Design review of the part built by this model. Coordinates are the model's own, in mm. A direction names the side the tool comes from. Coordinates: 2 decimals unless noted, no trailing zeros. Order: outer loops, then holes, each group sorted by start corner. A loop starts at its lowest first (then second) coordinate and runs counter-clockwise, first axis right, second up.
from build123d import *

# Parameters (mm, degrees)
SKETCH_1_R          = 1.6
EXTRUDE_1_DEPTH     = 3
SKETCH_2_R          = 1.6
CUT_EXTRUDE_1_DEPTH = 4
FILLET_1_R          = 3
SKETCH_4_R          = 1.6
CUT_EXTRUDE_2_DEPTH = 4
SKETCH_5_W          = 38
SKETCH_5_H          = 16
CUT_EXTRUDE_3_DEPTH = 4
FILLET_2_R          = 3


with BuildPart() as part:
    # 草图1 → 凸台-拉伸1 (new body)
    with BuildSketch(Plane.XY):
        Polygon((-40, 0), (-48, 25.544444444), (-48, 53.5), (5, 53.5), (5, 25.544444444), (0, 0), align=None)
        with Locations((-44, 49.5)):
            Circle(SKETCH_1_R, mode=Mode.SUBTRACT)
        with Locations((1, 49.5)):
            Circle(SKETCH_1_R, mode=Mode.SUBTRACT)
        with Locations((1, 27.5)):
            Circle(SKETCH_1_R, mode=Mode.SUBTRACT)
        with Locations((-44, 27.5)):
            Circle(SKETCH_1_R, mode=Mode.SUBTRACT)
    extrude(amount=EXTRUDE_1_DEPTH)

    # 草图2 → 切除-拉伸1 (cut, through all)
    with BuildSketch(Plane.XY.offset(3)):
        with Locations((-5, 3)):
            Circle(SKETCH_2_R)
        with Locations((-15, 3)):
            Circle(SKETCH_2_R)
        with Locations((-25, 3)):
            Circle(SKETCH_2_R)
        with Locations((-35, 3)):
            Circle(SKETCH_2_R)
    extrude(amount=-CUT_EXTRUDE_1_DEPTH, mode=Mode.SUBTRACT)

    # 圆角1
    fillet_1_edges = [part.edges().sort_by_distance(p)[0] for p in [
        (0, 0, 1.5),
        (-40, 0, 1.5),
        (-48, 25.544444444, 1.5),
        (-48, 53.5, 1.5),
        (5, 53.5, 1.5),
        (5, 25.544444444, 1.5),
    ]]
    fillet(fillet_1_edges, radius=FILLET_1_R)

    # 草图4 → 切除-拉伸2 (cut, through all)
    with BuildSketch(Plane.XY.offset(3)):
        with Locations((-21.5, 36.5)):
            Circle(SKETCH_4_R)
        with Locations((-33.5, 12.5)):
            Circle(SKETCH_4_R)
        with Locations((-21.5, 12.5)):
            Circle(SKETCH_4_R)
    extrude(amount=-CUT_EXTRUDE_2_DEPTH, mode=Mode.SUBTRACT)

    # 草图5 → 切除-拉伸3 (cut, through all)
    with BuildSketch(Plane(origin=(0, 0, 0), x_dir=(-1, 0, 0), z_dir=(0, 0, -1))):
        with Locations((21.5, 38.5)):
            Rectangle(SKETCH_5_W, SKETCH_5_H)
    extrude(amount=-CUT_EXTRUDE_3_DEPTH, mode=Mode.SUBTRACT)

    # 圆角2
    fillet_2_edges = [part.edges().sort_by_distance(p)[0] for p in [
        (-40.5, 46.5, 1.5),
        (-40.5, 30.5, 1.5),
        (-2.5, 30.5, 1.5),
        (-2.5, 46.5, 1.5),
    ]]
    fillet(fillet_2_edges, radius=FILLET_2_R)


solid = part.part
1. For faces 4 (the flat face through (-21, 27, 0)), 5 (the cylindrical face through (-39.64, 45.6, 1.52)), list the 3-axis set-ups (+Z, -Z, +X, -X, +Y, -Y) from which the entire face can be reached by the end or side of a thin tool; tool diameter is ignored.
2. Insertion check: pin 1 (3 mm diameter, centred on x = -25, y = 3, fed in from -Z). The pin has a flat end and moves straight along its axis. Give the tip position at first contact, or say it passes through.
3. To check wall thickness, follow line 1 (Y direction, x = -21.5, z = 1.2); line 2 (Y direction, x = -36, z = 2.3); line 3 (X direction, y = 36, z = 0.7). State the ranges of each line that lie inside material, in increasing order.
4. Add section B-B (x = -25). Give the boundary of the cut face in (y, z), and give its area (3 significant figures).
5. Mouldability with a two-part tool opening along Y and no side actions: class faces 1 (the cylindrical face through (-0.585, 0.666, 1.521)), 2 (the cylindrical face through (-3.4, 31.36, 1.52)), 3 (the flat face through (5, 38, 1)) as pulls with the +Y half, pulls with the -Y half, needs draft (parallel to the pull), parting line crosses it, or undercut.
6. Add section A-A (z = 1). State how many separate pieces and enclosed holes the cut face has, and give its area (3 significant figures).
Solution:
1. face 4: -Z, +X, -X, +Y, -Y
1. face 5: +Z, -Z
2. pin 1: passes through
3. line 1: y = 0 to 10.9, 14.1 to 30.5, 46.5 to 53.5
3. line 2: y = 0 to 1.75, 4.25 to 30.5, 46.5 to 53.5
3. line 3: x = -48 to -40.5, -2.5 to 5
4. outline: (0, 0) - (1.4, 0) - (1.4, 3) - (0, 3) - close; (4.6, 0) - (30.5, 0) - (30.5, 3) - (4.6, 3) - close; (46.5, 0) - (53.5, 0) - (53.5, 3) - (46.5, 3) - close
4. area: 103 mm2
5. face 1: pulls with the -Y half
5. face 2: undercut
5. face 3: needs draft
6. separate pieces: 1
6. enclosed holes: 11
6. area: 1,980 mm2
